Work out the finished part from the listing and answer in its coordinate system (mm). A direction names the side the tool comes from. Round coordinates to 2 decimals unless told otherwise and drop trailing zeros. Write each loop counter-clockwise with the first axis right and the second up, starting at its lowest first coordinate (ties: lowest second). Pieces come first, ordered by that corner, then holes. Notation, with made-up numbers: (-18, 72.5) - (-2, 72.5) arc R23 ccw to (-2, 88.5) - close; hole circle Ø1 at (15, -17). An arc over 180 degrees is marked (long way). Answer as a JSON object with one key per item and string values.
```python
from build123d import *

# Parameters (mm, degrees)
BOSS_EXTRUDE1_DEPTH = 3
BOSS_EXTRUDE2_DEPTH = 5
SKETCH3_R           = 5
SKETCH3_R_2         = 9
CUT_EXTRUDE1_DEPTH  = 3
SKETCH4_R           = 9
SKETCH4_R_2         = 8
BOSS_EXTRUDE3_DEPTH = 3
SKETCH4_3_R         = 6
SKETCH4_3_R_2       = 5
BOSS_EXTRUDE4_DEPTH = 3
SKETCH6_R           = 10.5
SKETCH6_R_2         = 9
BOSS_EXTRUDE5_DEPTH = 6
SKETCH7_R           = 10.5
SKETCH7_R_2         = 9
CUT_EXTRUDE2_DEPTH  = 1


with BuildPart() as part:
    # Sketch1 → Boss-Extrude1 (new body)
    with BuildSketch(Plane(origin=(0, 0, 0), x_dir=(1, 0, 0), z_dir=(0, 1, 0))):
        with BuildLine():
            Line((-43, 25.514701644), (-43, -25.514701644))
            ThreePointArc((-43, -25.514701644), (-37.211637523, -33.396018219), (-30, -40))
            Line((-30, -40), (-10, -40))
            Line((-10, -40), (-10, -48.989794856))
            ThreePointArc((-10, -48.989794856), (45.716299059, 20.248950598), (-43, 25.514701644))
        make_face()
    extrude(amount=BOSS_EXTRUDE1_DEPTH)

    # Sketch2 → Boss-Extrude2 (add)
    with BuildSketch(Plane.XZ):
        with BuildLine():
            Line((-40.978122, 24.995870006), (-40.978122, -24.995870006))
            ThreePointArc((-40.978122, -24.995870006), (-26.914721681, -39.744153744), (-8, -47.328638265))
            Line((-8, -47.328638265), (-8, -45.299006612))
            ThreePointArc((-8, -45.299006612), (-25.702922785, -38.149177715), (-38.978122, -24.427566505))
            Line((-38.978122, -24.427566505), (-38.978122, 24.427566505))
            ThreePointArc((-38.978122, 24.427566505), (-34.298477795, 30.653130687), (-28.635642127, 36))
            Line((-28.635642127, 36), (-8, 36))
            Line((-8, 36), (-8, 38))
            Line((-8, 38), (-29.325756597, 38))
            ThreePointArc((-29.325756597, 38), (-35.748226329, 32.032238672), (-40.978122, 24.995870006))
        make_face()
        with BuildLine():
            Line((-6, 45.607017004), (-6, 47.623523599))
            ThreePointArc((-6, 47.623523599), (-4.003501138, 47.832750064), (-2, 47.958315233))
            Line((-2, 47.958315233), (-2, 45.956501172))
            ThreePointArc((-2, 45.956501172), (-4.00381503, 45.825423786), (-6, 45.607017004))
        make_face()
        with BuildLine():
            Line((-6, -45.607017004), (-6, -47.623523599))
            ThreePointArc((-6, -47.623523599), (-4.003501138, -47.832750064), (-2, -47.958315233))
            Line((-2, -47.958315233), (-2, -45.956501172))
            ThreePointArc((-2, -45.956501172), (-4.00381503, -45.825423786), (-6, -45.607017004))
        make_face()
        with BuildLine():
            Line((0, 46), (0, 48))
            ThreePointArc((0, 48), (48, 0), (0, -48))
            Line((0, -48), (0, -46))
            ThreePointArc((0, -46), (46, 0), (0, 46))
        make_face()
    extrude(amount=BOSS_EXTRUDE2_DEPTH)

    # Sketch3 → Cut-Extrude1 (cut)
    with BuildSketch(Plane.XZ):
        with Locations((25, 0)):
            Circle(SKETCH3_R)
        with Locations((15, 24)):
            Circle(SKETCH3_R_2)
    extrude(amount=-CUT_EXTRUDE1_DEPTH, mode=Mode.SUBTRACT)

    # Sketch4 → Boss-Extrude3 (add)
    with BuildSketch(Plane.XZ):
        with Locations((25, 0)):
            Circle(SKETCH4_R)
        with Locations((25, 0)):
            Circle(SKETCH4_R_2, mode=Mode.SUBTRACT)
    extrude(amount=BOSS_EXTRUDE3_DEPTH)

    # Sketch4_3 → Boss-Extrude4 (add)
    with BuildSketch(Plane.XZ):
        with Locations((25, 0)):
            Circle(SKETCH4_3_R)
        with Locations((25, 0)):
            Circle(SKETCH4_3_R_2, mode=Mode.SUBTRACT)
    extrude(amount=BOSS_EXTRUDE4_DEPTH)

    # Sketch6 → Boss-Extrude5 (add)
    with BuildSketch(Plane.XZ):
        with Locations((15, 24)):
            Circle(SKETCH6_R)
        with Locations((15, 24)):
            Circle(SKETCH6_R_2, mode=Mode.SUBTRACT)
    extrude(amount=BOSS_EXTRUDE5_DEPTH)

    # Sketch7 → Cut-Extrude2 (cut)
    with BuildSketch(Plane(origin=(0, 3, 0), x_dir=(1, 0, 0), z_dir=(0, 1, 0))):
        with Locations((15, -24)):
            Circle(SKETCH7_R)
        with Locations((15, -24)):
            Circle(SKETCH7_R_2, mode=Mode.SUBTRACT)
    extrude(amount=-CUT_EXTRUDE2_DEPTH, mode=Mode.SUBTRACT)


solid = part.part
```
Item 1: Consider line 1 along Y through (x, z) = (23.5, 20); line 2 along Y through (x, z) = (-20, -43); line 3 along Z through (x, y) = (13, 0.25). Determine where each line is inside the solid, lowest interval first.
Results found:
{"line 1": "-6 to 2", "line 2": "-5 to 3", "line 3": "-48.28 to 15.23, 32.77 to 48.28"}
Item 2: A cutting plane is placed at B-B (z = -18). Write down the section's boundary in (x, y).
Results found:
{"outline": "(-43, 0) - (-40.98, 0) - (-40.98, -5) - (-38.98, -5) - (-38.98, 0) - (42.33, 0) - (42.33, -5) - (44.5, -5) - (44.5, 0) - (46.65, 0) - (46.65, 3) - (-43, 3) - close"}
Item 3: For faces 4 (the cylindrical face through (20.24, -1.48, -3.65)), 5 (the cylindrical face through (-4.03, -2.46, -47.83)), 6 (the cylindrical face through (-35.67, -2.46, 32.12)), determine the directions among +Z, -Z, +X, -X, +Y, -Y from which every point of the face is accessible in a straight line to the end or side of a thin tool.
Results found:
{"face 4": "-Y", "face 5": "-Z, -X, -Y", "face 6": "+Z, -X, -Y"}
Item 4: A cutting plane is placed at D-D (z = 0). Write down the section's boundary in (x, y), and give its area (3 significant figures).
Results found:
{"outline": "(-43, 0) - (-40.98, 0) - (-40.98, -5) - (-38.98, -5) - (-38.98, 0) - (16, 0) - (16, -3) - (17, -3) - (17, 0) - (19, 0) - (19, -3) - (20, -3) - (20, 3) - (-43, 3) - close; (30, -3) - (31, -3) - (31, 0) - (33, 0) - (33, -3) - (34, -3) - (34, 0) - (46, 0) - (46, -5) - (48, -5) - (48, 0) - (50, 0) - (50, 3) - (30, 3) - close", "area": "281 mm²"}
Item 5: A cutting plane is placed at C-C (x = -27.5). Write down the section's boundary in (y, z), and give its area (3 significant figures).
Results found:
{"outline": "(-5, -39.34) - (0, -39.34) - (0, -41.76) - (3, -41.76) - (3, 40) - (0, 40) - (0, 38) - (-5, 38) - (-5, 36) - (0, 36) - (0, -36.87) - (-5, -36.87) - close", "area": "268 mm²"}
Item 6: A cutting plane is placed at A-A (z = 19.5). Write down the section's boundary in (x, y).
Results found:
{"outline": "(-43, 0) - (-40.98, 0) - (-40.98, -5) - (-38.98, -5) - (-38.98, 0) - (5.51, 0) - (5.51, -6) - (7.21, -6) - (7.21, 2) - (5.51, 2) - (5.51, 3) - (-43, 3) - close; (22.79, -6) - (24.49, -6) - (24.49, 0) - (41.66, 0) - (41.66, -5) - (43.86, -5) - (43.86, 0) - (46.04, 0) - (46.04, 3) - (24.49, 3) - (24.49, 2) - (22.79, 2) - close"}
Item 7: Determine the mould class of faces 1 (the cylindrical face through (47.99, -2.46, 1.06)), 2 (the flat face through (-40.978, -2, 0)), 3 (the cylindrical face through (23.584, -1.944, 26.703)) for opening direction Z: pulls with the +Z half, pulls with the -Z half, needs draft (parallel to the pull), parting line crosses it, or undercut.
Results found:
{"face 1": "parting line crosses it", "face 2": "needs draft", "face 3": "undercut"}
Item 8: Each of these flat-tipped pins is pushed along its axis until it touches: P1, Ø0.9, axis at y = 1, z = 46.5, coming from the -X side; P2, Ø8, axis at x = 25, z = 0, coming from the +Y side; P3, Ø20, axis at x = 28.5, z = 1, coming from the -Y side; P4, Ø17, axis at x = 10, z = 29, coming from the +Y side. Where does it stop, or does it pass through?
Results found:
{"P1": "x = -10", "P2": "through", "P3": "y = -3", "P4": "y = 3"}
